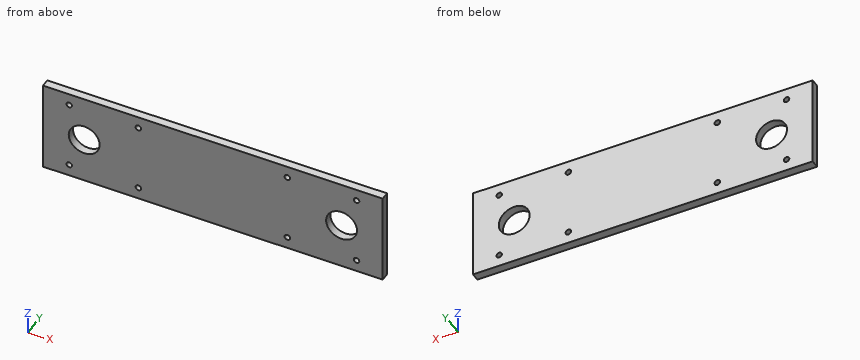
from build123d import *

# Parameters (mm, degrees)
SKETCH1_W           = 330
SKETCH1_H           = 91
BOSS_EXTRUDE2_DEPTH = 8
SKETCH4_R           = 15
SKETCH4_R_2         = 2.7
CUT_EXTRUDE4_DEPTH  = 8


with BuildPart() as part:
    # Sketch1 → Boss-Extrude2 (new body)
    with BuildSketch(Plane(origin=(0, 0, 0), x_dir=(1, 0, 0), z_dir=(0, 1, 0))):
        Rectangle(SKETCH1_W, SKETCH1_H)
    extrude(amount=BOSS_EXTRUDE2_DEPTH)

    # Sketch4 → Cut-Extrude4 (cut)
    with BuildSketch(Plane(origin=(0, 8, 0), x_dir=(1, 0, 0), z_dir=(0, 1, 0))):
        with Locations(Location((125, 0, 0), (0, 0, 270))):
            Circle(SKETCH4_R)
        with Locations(Location((-125, 0, 0), (0, 0, 270))):
            Circle(SKETCH4_R)
        with Locations(Location((-139.55, 33.59, 0), (0, 0, 270))):
            Circle(SKETCH4_R_2)
        with Locations(Location((-139.55, -33.59, 0), (0, 0, 270))):
            Circle(SKETCH4_R_2)
        with Locations(Location((-72.37, -33.59, 0), (0, 0, 270))):
            Circle(SKETCH4_R_2)
        with Locations(Location((-72.37, 33.59, 0), (0, 0, 270))):
            Circle(SKETCH4_R_2)
        with Locations(Location((139.55, -33.59, 0), (0, 0, 90))):
            Circle(SKETCH4_R_2)
        with Locations(Location((72.37, -33.59, 0), (0, 0, 90))):
            Circle(SKETCH4_R_2)
        with Locations(Location((72.37, 33.59, 0), (0, 0, 90))):
            Circle(SKETCH4_R_2)
        with Locations(Location((139.55, 33.59, 0), (0, 0, 90))):
            Circle(SKETCH4_R_2)
    extrude(amount=-CUT_EXTRUDE4_DEPTH, mode=Mode.SUBTRACT)


solid = part.part
Source: CAD feature listing. Evaluate the final solid. Frame: model axes, mm. Round coordinates to 2 decimals unless told otherwise and drop trailing zeros. Order: outer loops, then holes, each group sorted by start corner. A loop starts at its lowest first (then second) coordinate and runs counter-clockwise, first axis right, second up. Notation, with made-up numbers: (58, -40) - (81, -40) arc R20 ccw to (81, -24) - close; hole circle Ø11 at (36.25, 33.25). An arc over 180 degrees is marked (long way). Use a Markdown table: item, result. Add a question column.
1. Section query C-C (y = 5.75). Give the number of separate pieces and of enclosed holes in the cut face, then the cut area to 3 significant figures.
2. Section query B-B (x = 131). Return the cut outline in (y, z), then the cut area to 3 significant figures.
3. Line query: probe 1 along X at (y, z) = (6.75, 0); probe 2 along X at (y, z) = (5.5, -33.59); probe 3 along Z at (x, y) = (72.37, 2). Output: solid intervals per line, ascending.
4. Section query A-A (z = 0). Return the cut outline in (x, y), then the cut area to 3 significant figures.
5. First-contact query: pin 1 (3 mm diameter, centred on x = 139.55, z = -33.59, fed in from +Y). Flat tip, straight axial feed; report the tip coordinate or a pass-through.
Derived:
| question | item | result |
|---|---|---|
| 1 | separate pieces | 1 |
| 1 | enclosed holes | 10 |
| 1 | area | 28,400 mm2 |
| 2 | outline | (0, -45.5) - (8, -45.5) - (8, -13.75) - (0, -13.75) - close; (0, 13.75) - (8, 13.75) - (8, 45.5) - (0, 45.5) - close |
| 2 | area | 508 mm2 |
| 3 | probe 1 | -165 to -140, -110 to 110, 140 to 165 |
| 3 | probe 2 | -165 to -142.25, -136.85 to -75.07, -69.67 to 69.67, 75.07 to 136.85, 142.25 to 165 |
| 3 | probe 3 | -45.5 to -36.29, -30.89 to 30.89, 36.29 to 45.5 |
| 4 | outline | (-165, 0) - (-140, 0) - (-140, 8) - (-165, 8) - close; (-110, 0) - (110, 0) - (110, 8) - (-110, 8) - close; (140, 0) - (165, 0) - (165, 8) - (140, 8) - close |
| 4 | area | 2,160 mm2 |
| 5 | pin 1 | through |
